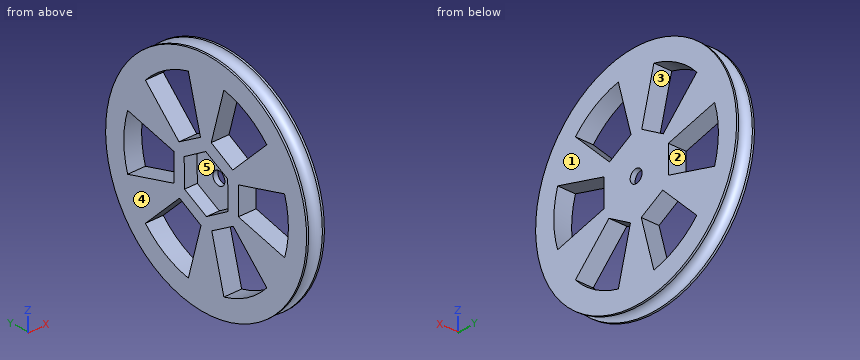
```python
from build123d import *

# Parameters (mm, degrees)
SKETCH2_W          = 0.508
SKETCH2_H          = 27.94
CUT_EXTRUDE1_REACH = 41.774
SKETCH3_R          = 1.651
CIRPATTERN1_COUNT  = 6
SKETCH3_3_R        = 1.651
CUT_EXTRUDE2_DEPTH = 3.2766


with BuildPart() as part:
    # Sketch2 → Revolve1 (revolve)
    with BuildSketch(Plane.XY, mode=Mode.PRIVATE) as revolve1_sk:
        with Locations((-0.254, 13.97)):
            Rectangle(SKETCH2_W, SKETCH2_H)
        with BuildLine():
            ThreePointArc((0, 27.94), (1.7653, 26.1747), (3.5306, 27.94))
            Line((3.5306, 27.94), (3.5306, 0))
            Line((3.5306, 0), (0, 0))
            Line((0, 0), (0, 27.94))
        make_face()
        with Locations((3.7846, 13.97)):
            Rectangle(SKETCH2_W, SKETCH2_H)
    revolve(revolve1_sk.sketch.rotate(Axis((0, 0, 0), (1, 0, 0)), 90), axis=Axis((0, 0, 0), (1, 0, 0)))

    # Sketch3 → Cut-Extrude1 (cut, up to next)
    with BuildSketch(Plane(origin=(-0.508, 0, 0), x_dir=(0, 0, -1), z_dir=(1, 0, 0)), mode=Mode.PRIVATE) as cut_extrude1_sk1:
        with BuildLine():
            ThreePointArc((6.891742224, 21.816499024), (0, 22.879155153), (-6.891742224, 21.816499024))
            Line((-6.891742224, 21.816499024), (-3.362938361, 8.966871047))
            Line((-3.362938361, 8.966871047), (3.528803863, 8.966871047))
            Line((3.528803863, 8.966871047), (6.891742224, 21.816499024))
        make_face()
    cut_extrude1_tool1 = extrude(cut_extrude1_sk1.sketch, amount=CUT_EXTRUDE1_REACH, mode=Mode.PRIVATE) & part.part
    # Sketch3 → Cut-Extrude1 (cut, up to next)
    with BuildSketch(Plane(origin=(-0.508, 0, 0), x_dir=(0, 0, -1), z_dir=(1, 0, 0)), mode=Mode.PRIVATE) as cut_extrude1_sk2:
        with Locations(Location((0, 0, 0), (0, 0, 180))):
            Circle(SKETCH3_R)
    cut_extrude1_tool2 = extrude(cut_extrude1_sk2.sketch, amount=CUT_EXTRUDE1_REACH, mode=Mode.PRIVATE) & part.part
    cut_extrude1_1 = cut_extrude1_tool1.solids().sort_by_distance((-0.508, 16.527641, -0.034324))[0]
    add(cut_extrude1_1, mode=Mode.SUBTRACT)
    cut_extrude1_2 = cut_extrude1_tool2.solids().sort_by_distance((-0.508, 0, 0))[0]
    add(cut_extrude1_2, mode=Mode.SUBTRACT)
    cut_extrude1 = cut_extrude1_1 + cut_extrude1_2  # Cut-Extrude1 as one shape, for the pattern or mirror that repeats it

    # CirPattern1: Cut-Extrude1 ×6 about axis
    cirpattern1_axis = Axis((0, 0, 0), (1, 0, 0))
    for i in range(1, CIRPATTERN1_COUNT):
        add(cut_extrude1.rotate(cirpattern1_axis, i * 360 / CIRPATTERN1_COUNT), mode=Mode.SUBTRACT)

    # Sketch3<3> → Cut-Extrude2 (cut)
    with BuildSketch(Plane(origin=(-0.508, 0, 0), x_dir=(0, 0, -1), z_dir=(1, 0, 0))):
        Polygon((6.984325773, -0.097048964), (3.576209755, 6.000079065), (-3.408116018, 6.09712803), (-6.984325773, 0.097048964), (-3.576209755, -6.000079065), (3.408116018, -6.09712803), align=None)
        Circle(SKETCH3_3_R, mode=Mode.SUBTRACT)
    extrude(amount=CUT_EXTRUDE2_DEPTH, mode=Mode.SUBTRACT)


solid = part.part
```
Part model, mm, in its own coordinate system. Face numbers are marked on the shaded views. A direction names the side the tool comes from. Give positions to 0.01 mm unless a question says otherwise; leave off trailing zeros. Order: outer loops, then holes, each group sorted by start corner. A loop starts at its lowest first (then second) coordinate and runs counter-clockwise, first axis right, second up. Notation, with made-up numbers: M -20,-29.75 L 2,-29.75 A22 ccw 2,-23.75 Z; hole C 78,55.25 d2. An arc over 180 degrees is marked long. Use a Markdown table: item, result. Add a question column.
(1) Mould opens along Z. For the marked faces 1 and 2 say: +Z half, -Z half, draft (parallel to the pull), parting line (faces both ways), or undercut.
(2) 3-axis set-ups, long thin cutter, end or side, ignore diameter. For the marked faces 3, 4 and 5: which of +Z, -Z, +X, -X, +Y, -Y reach the whole face in a straight line?
(3) Probe line 1 along Y through (x, z) = (3.6, 0); line 2 along Z through (x, y) = (1.8, 14.5); line 3 along Y through (x, z) = (1.9, -0.5). List the from-to ranges inside material, lowest first. Write a range as [from, to].
(4) Drop flat-ended pins along their axis: P1, Ø1.5, axis at x = 1, y = -16.5, coming from the -Z side; P2, Ø3.5, axis at y = 1.5, z = -2.5, coming from the -X side; P3, Ø1.4, axis at x = 1.5, z = 0, coming from the -Y side. Give the stop position or say it passes through.
(5) Saw through at A-A, the plane z = 0. Give the cut face in (x, y).
(6) Saw through at B-B, the plane x = 1.8. Give the number of separate pieces and of enclosed holes in the cut face, and give its area (3 significant figures).
Answer key:
| question | item | result |
|---|---|---|
| 1 | face 1 | draft |
| 1 | face 2 | undercut |
| 2 | face 3 | +X, -X |
| 2 | face 4 | +Z, -Z, -X, +Y, -Y |
| 2 | face 5 | -X |
| 3 | line 1 | [-27.94, -22.88], [-8.97, -1.65], [1.65, 8.97], [22.88, 27.94] |
| 3 | line 2 | [-21.79, -17.7], [-13.1, -4.98], [4.88, 13.04], [17.7, 21.79] |
| 3 | line 3 | [-26.18, -22.87], [-8.97, -6.06], [6.04, 8.97], [22.87, 26.18] |
| 4 | P1 | z = -21.52 |
| 4 | P2 | x = 2.77 |
| 4 | P3 | y = -26.46 |
| 5 | outline | M -0.51,-27.94 L 0,-27.94 A1.77 cw 3.53,-27.94 L 4.04,-27.94 L 4.04,-22.88 L -0.51,-22.88 Z; M -0.51,-8.97 L 4.04,-8.97 L 4.04,-1.65 L 2.77,-1.65 L 2.77,-6.05 L -0.51,-6.05 Z; M -0.51,6.05 L 2.77,6.05 L 2.77,1.65 L 4.04,1.65 L 4.04,8.97 L -0.51,8.97 Z; M -0.51,22.88 L 4.04,22.88 L 4.04,27.94 L 3.53,27.94 A1.77 cw 0,27.94 L -0.51,27.94 Z |
| 6 | separate pieces | 1 |
| 6 | enclosed holes | 7 |
| 6 | area | 1,170 mm^2 |
